Verification items for the finished model (mm, model axes). Face numbers are marked on the shaded views. Round coordinates to 2 decimals unless told otherwise and drop trailing zeros. Write each loop counter-clockwise with the first axis right and the second up, starting at its lowest first coordinate (ties: lowest second). Pieces come first, ordered by that corner, then holes. Notation, with made-up numbers: M 28,-5.75 L 70,-5.75 A19 ccw 70,11.25 Z; hole C -36,-11 d4. An arc over 180 degrees is marked long. One line per question, with ' | ' between items.
from build123d import *

# Parameters (mm, degrees)
SKETCH1_R           = 2.5
SKETCH1_R_2         = 1.5
BOSS_EXTRUDE1_DEPTH = 3
BOSS_EXTRUDE2_START = -0.75
BOSS_EXTRUDE2_DEPTH = 0.75


with BuildPart() as part:
    # Sketch1 → Boss-Extrude1 (new body)
    with BuildSketch(Plane(origin=(0, 0, 0), x_dir=(0, 0, -1), z_dir=(1, 0, 0))):
        Circle(SKETCH1_R)
        Circle(SKETCH1_R_2, mode=Mode.SUBTRACT)
    extrude(amount=BOSS_EXTRUDE1_DEPTH)

    # Sketch2 → Boss-Extrude2 (add)
    with BuildSketch(Plane(origin=(3, 0, 0), x_dir=(0, 0, -1), z_dir=(1, 0, 0)).offset(BOSS_EXTRUDE2_START)):
        with BuildLine():
            Line((-1.5, 2), (-1.5, 12.632795692))
            ThreePointArc((-1.5, 12.632795692), (0, 14.132795692), (1.5, 12.632795692))
            Line((1.5, 12.632795692), (1.5, 2))
            ThreePointArc((1.5, 2), (0, -2.5), (-1.5, 2))
        make_face()
    extrude(amount=BOSS_EXTRUDE2_DEPTH)


solid = part.part
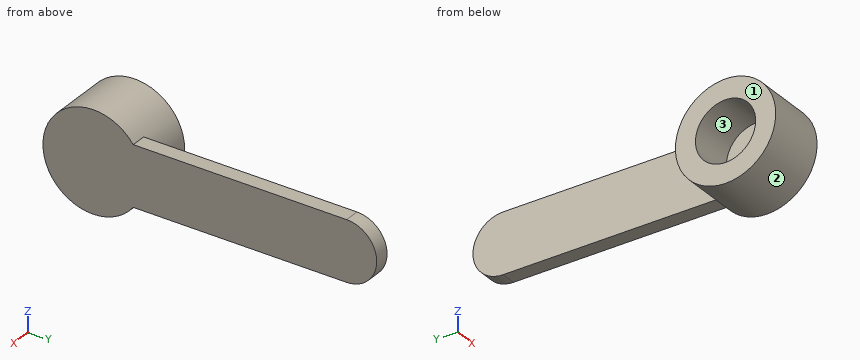
1. Go/stop test with flat-tipped pins: P1, Ø3, axis at y = 8, z = -1, coming from the -X side; P2, Ø0.8, axis at x = 3, y = 6.5, coming from the +Z side. Record where each tip stops, or that it passes through.
Results:
P1: stops at x = 2.25 | P2: stops at z = 1.5
2. Section check C-C, the plane x = 0.5. Record the cut outline in (y, z).
Results:
outline: C 0,0 d5; hole C 0,0 d3
3. Mould release check, pull along Y, two halves, no side actions. Record for the marked faces 1, 2 and 3: pulls with the +Y half, pulls with the -Y half, needs draft (parallel to the pull), parting line crosses it, or undercut.
Results:
face 1: needs draft | face 2: parting line crosses it | face 3: undercut
4. Thickness scan on line 1 (Y direction, x = 1.2, z = 0); line 2 (X direction, y = 8.75, z = -1). Record the ranges inside material, lowest first.
Results:
line 1: y = -2.5 to -1.5, 1.5 to 2.5 | line 2: x = 2.25 to 3
5. Section check B-B, the plane z = 0. Record the cut outline in (x, y), then the cut area to 3 significant figures.
Results:
outline: M 0,-2.5 L 3,-2.5 L 3,14.13 L 2.25,14.13 L 2.25,2.5 L 0,2.5 L 0,1.5 L 2.25,1.5 L 2.25,-1.5 L 0,-1.5 Z | area: 17.0 mm2
6. Section check D-D, the plane y = 8.75. Record the cut outline in (x, z), then the cut area to 3 significant figures.
Results:
outline: M 2.25,-1.5 L 3,-1.5 L 3,1.5 L 2.25,1.5 Z | area: 2.25 mm2
7. Section check A-A, the plane y = 0. Record the cut outline in (x, z), then the cut area to 3 significant figures.
Results:
outline: M 0,-2.5 L 3,-2.5 L 3,2.5 L 0,2.5 L 0,1.5 L 2.25,1.5 L 2.25,-1.5 L 0,-1.5 Z | area: 8.25 mm2
